from build123d import *

# Parameters (mm, degrees)
F0_R     = 63.5
F1_DEPTH = 3.429
F2_SIZE  = 19.05


with BuildPart() as f1:
    # F0 (on Front) → F1 (new body)
    with BuildSketch(Plane.XZ):
        Polygon((-200.025, -110.871), (200.025, -110.871), (200.025, 110.871), (15.0876, 110.871), (15.0876, 16.129), (10.3124, 16.129), (10.3124, 110.871), (-200.025, 110.871), align=None)
        with Locations((-94.8563, 0)):
            Circle(F0_R, mode=Mode.SUBTRACT)
        with Locations((107.5563, 0)):
            Circle(F0_R, mode=Mode.SUBTRACT)
    extrude(amount=F1_DEPTH)

    # F2
    f2_edges = [f1.edges().sort_by_distance(p)[0] for p in [
        (-200.025, -1.7145, 110.871),
        (10.3124, -1.7145, 110.871),
        (15.0876, -1.7145, 110.871),
        (200.025, -1.7145, 110.871),
        (200.025, -1.7145, -110.871),
        (-200.025, -1.7145, -110.871),
    ]]
    chamfer(f2_edges, length=F2_SIZE)


solid = f1.part
Here's how the part is built. I have some questions about the finished solid (model axes, mm). A direction names the side the tool comes from. Coordinates: 2 decimals unless noted, no trailing zeros. Write each loop counter-clockwise with the first axis right and the second up, starting at its lowest first coordinate (ties: lowest second). Pieces come first, ordered by that corner, then holes. Notation, with made-up numbers: (51, 54.5) - (96, 54.5) arc R13 cw to (96, 72.5) - close; hole circle Ø3 at (-32.5, -35). An arc over 180 degrees is marked (long way). Use one line per item in the form item = value.
1) Thinking about a two-plate mould opening in Z: for faces 3 (the cylindrical face through (168.124, -1.69, 19.074)), 4 (the flat face through (-3, -3.429, 2)), 5 (the flat face through (190.633, -1.69, -101.213)), which applies, released by +Z, released by -Z, zero draft, split by the parting line, or undercut?
Solved:
face_3 = undercut
face_4 = zero draft
face_5 = released by -Z
2) Suppose I cut it at C-C, the plane z = 41.5. Write out the boundary of the cut face in (x, y) (3 decimals).
Solved:
outline = (-200.025, -3.429) - (-142.919, -3.429) - (-142.919, 0) - (-200.025, 0) - close; (-46.794, -3.429) - (10.312, -3.429) - (10.312, 0) - (-46.794, 0) - close; (15.088, -3.429) - (59.494, -3.429) - (59.494, 0) - (15.088, 0) - close; (155.619, -3.429) - (200.025, -3.429) - (200.025, 0) - (155.619, 0) - close
3) I need wall thicknesses on line 1 (X direction, y = -1.35, z = 2) (3 decimals); line 2 (X direction, y = -3.05, z = -38.5) (3 decimals); line 3 (X direction, y = -1.9, z = 70.5) (3 decimals). Which ranges of each line are inside material? Lowest first, please.
Solved:
line_1 = -200.025 to -158.325, -31.388 to 44.088, 171.025 to 200.025
line_2 = -200.025 to -145.354, -44.359 to 57.059, 158.054 to 200.025
line_3 = -200.025 to 10.312, 15.088 to 200.025
4) On a 3-axis mill with a long thin cutter (end or side, diameter ignored), from which of +Z, -Z, +X, -X, +Y, -Y can I reach the whole of each face in a straight line? I mean faces 1 (the flat face through (-190.367, -1.69, 101.479)), 2 (the flat face through (24.479, -1.69, 101.213)). Say none if no direction works.
Solved:
face_1 = +Z, -X, +Y, -Y
face_2 = +Z, +Y, -Y
5) Suppose I cut it at B-B, the plane y = -2.85. Write out the boundary of the cut face in (x, z) (3 decimals).
Solved:
outline = (-200.025, -91.821) - (-180.975, -110.871) - (180.975, -110.871) - (200.025, -91.821) - (200.025, 91.821) - (180.975, 110.871) - (34.138, 110.871) - (15.088, 91.821) - (15.088, 16.129) - (10.312, 16.129) - (10.312, 91.821) - (-8.738, 110.871) - (-180.975, 110.871) - (-200.025, 91.821) - close; hole circle Ø127 at (-94.856, 0); hole circle Ø127 at (107.556, 0)
6) Suppose I cut it at A-A, the plane z = 0. Write out the boundary of the cut face in (x, y) (3 decimals).
Solved:
outline = (-200.025, -3.429) - (-158.356, -3.429) - (-158.356, 0) - (-200.025, 0) - close; (-31.356, -3.429) - (44.056, -3.429) - (44.056, 0) - (-31.356, 0) - close; (171.056, -3.429) - (200.025, -3.429) - (200.025, 0) - (171.056, 0) - close
7) Suppose I cut it at D-D, the plane z = -50.5. Write out the boundary of the cut face in (x, y) (3 decimals).
Solved:
outline = (-200.025, -3.429) - (-133.353, -3.429) - (-133.353, 0) - (-200.025, 0) - close; (-56.36, -3.429) - (69.06, -3.429) - (69.06, 0) - (-56.36, 0) - close; (146.053, -3.429) - (200.025, -3.429) - (200.025, 0) - (146.053, 0) - close
8) I'm going to push a flat-ended pin straight in: P1, Ø1, axis at x = 13, y = -1.5, coming from the +Z side. Where does the tip first touch, or does it pass through?
Solved:
P1 = 16.13
